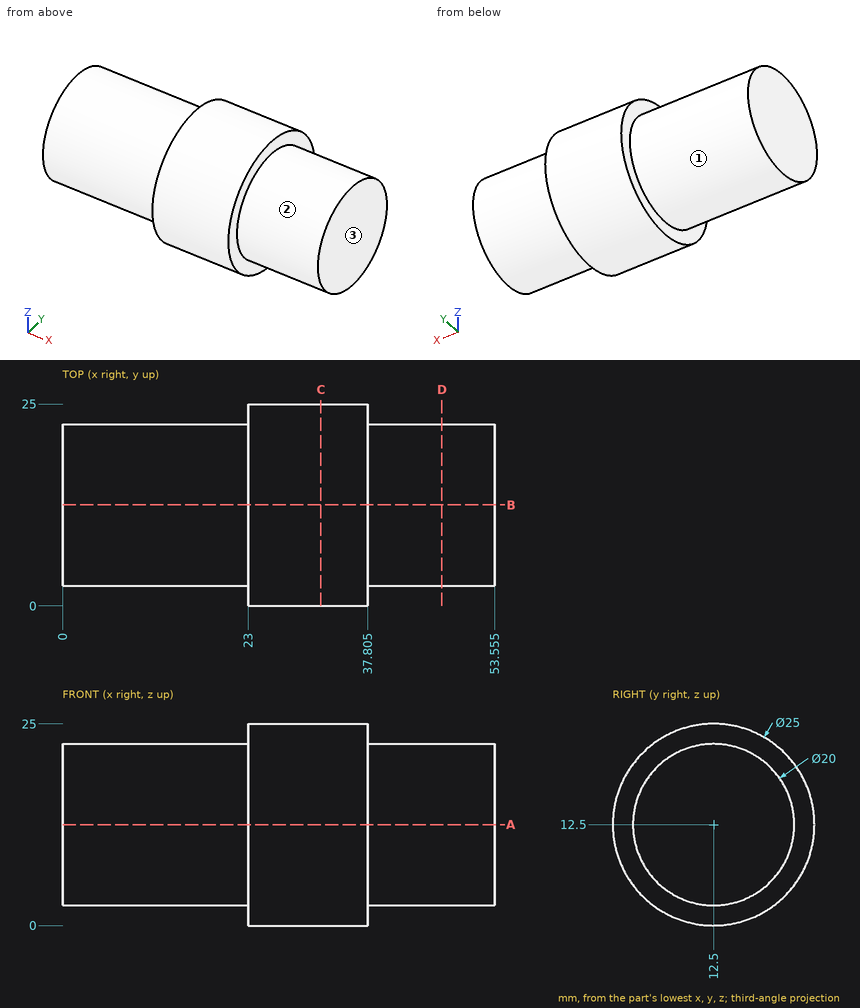
For this review, use the dimensioned drawing (mm, ordinates from the lowest corner) and the shaded views. A direction names the side the tool comes from. Give positions to 0.01 mm unless a question says otherwise; leave off trailing zeros. Loops run counter-clockwise (first coordinate to the right, second up) from the corner with the lowest first, then second, coordinate; pieces in that order, holes last. Notation, with made-up numbers: (41.5, 47) -> (45.5, 47) arc R15 ccw to (45.5, 56) -> close; hole circle Ø8 at (58, -31.5). An arc over 180 degrees is marked (long way). Use CSV: the item, a comma, the result in double quotes.
1. Consider section C-C, the plane x = 32. Write out the cut boundary in (y, z), then the cut area to 3 significant figures.
Result:
outline,"circle Ø25 at (12.5, 12.5)"
area,"491 mm²"
2. Consider section A-A, the plane z = 12.5. Write out the cut boundary in (x, y) (3 decimals).
Result:
outline,"(0, 2.5) -> (23, 2.5) -> (23, 0) -> (37.805, 0) -> (37.805, 2.5) -> (53.555, 2.5) -> (53.555, 22.5) -> (37.805, 22.5) -> (37.805, 25) -> (23, 25) -> (23, 22.5) -> (0, 22.5) -> close"
3. To check wall thickness, follow probe 1 along X at (y, z) = (4.5, 4.5) (3 decimals); probe 2 along Z at (x, y) = (34, 20); probe 3 along Y at (x, z) = (13.5, 7.5). State the ranges of each line that lie inside material, in increasing order. Write a range as from..to.
Result:
probe 1,"x = 23..37.805"
probe 2,"z = 2.5..22.5"
probe 3,"y = 3.84..21.16"
4. For P1, Ø4, axis at x = 40.5, y = 22.5, coming from the +Z side; P2, Ø12, axis at x = 5.5, y = 13, coming from the +Z side; P3, Ø12, axis at x = 17.5, z = 19, coming from the -Y side, all flat-tipped, find the tip position at first contact; note any pin that passes through.
Result:
P1,"stops at z = 18.5"
P2,"stops at z = 22.5"
P3,"stops at y = 0.69"
5. Machinability: for the marked faces 1, 2 and 3, which of the approach directions +Z, -Z, +X, -X, +Y, -Y give a long, thin tool a straight path to every point of the face, cutting with its end or side? Answer none if there is none.
Result:
face 1,"-X"
face 2,"+X"
face 3,"+Z, -Z, +X, +Y, -Y"
6. Consider section D-D, the plane x = 47. Write out the cut boundary in (y, z), then the cut area to 3 significant figures.
Result:
outline,"circle Ø20 at (12.5, 12.5)"
area,"314 mm²"
